from build123d import *

# Parameters (mm, degrees)
BOSS_EXTRUDE1_DEPTH = 50.1015


with BuildPart() as part:
    # Sketch1 → Boss-Extrude1 (new, symmetric)
    with BuildSketch(Plane(origin=(0, 0, 0), x_dir=(1, 0, 0), z_dir=(0, 1, 0))):
        Polygon((2.886751346, 0), (1.443375673, 2.5), (-1.443375673, 2.5), (-2.886751346, 0), (-1.443375673, -2.5), (1.443375673, -2.5), align=None)
    extrude(amount=BOSS_EXTRUDE1_DEPTH, both=True)

    # Sketch3 → M3x0.5 Tapped Hole1 (revolve, cut)
    with BuildSketch(Plane(origin=(0, 50.1015, 0), x_dir=(0, 0, 1), z_dir=(1, 0, 0))):
        Polygon((0, 0), (0, 10.276075774), (1.25, 9.525), (1.25, 0), align=None)
    m3x0_5_tapped_hole1 = revolve(axis=Axis((0, 56.4515, 0), (0, -1, 0)), mode=Mode.SUBTRACT)

    # Mirror1: M3x0.5 Tapped Hole1 across plane
    add(m3x0_5_tapped_hole1.mirror(Plane.ZX), mode=Mode.SUBTRACT)


solid = part.part
Work out the finished part from the listing and answer in its coordinate system (mm). A direction names the side the tool comes from. Round coordinates to 2 decimals unless told otherwise and drop trailing zeros. Write each loop counter-clockwise with the first axis right and the second up, starting at its lowest first coordinate (ties: lowest second). Pieces come first, ordered by that corner, then holes. Notation, with made-up numbers: (26.25, 78.5) -> (60.25, 78.5) arc R15 cw to (60.25, 88.5) -> close; hole circle Ø1 at (52, 11). An arc over 180 degrees is marked (long way). Answer as CSV lines item,"result". Start each with the question number.
(1) The part is cut by section A-A, the plane y = 44. Give the vertices of the cut face in (x, z).
(2) The mould has two halves that part along Z. Classify faces 1 (the conical face through (0.212, 39.956, -0.047)), 2 (the cylindrical face through (1.22, 45.41, -0.27)), 3 (the flat face through (2.175, 0.701, -1.233)), 4 (the flat face through (0, 1, 2.5)): +Z half, -Z half, draft (parallel to the pull), parting line (faces both ways), or undercut.
(3) Each of these flat-tipped pins is pushed along its axis until it touches: pin 1 (3 mm diameter, centred on x = 0, z = 0, fed in from +Y); pin 2 (1 mm diameter, centred on y = 33.5, z = -1, fed in from -X); pin 3 (1 mm diameter, centred on x = -2, y = 1, fed in from -Z). Where does it stop, or does it pass through?
(4) A tool of negligible diameter and unlimited length cuts with its end or side. For faces 5 (the flat face through (2.155, 0.701, 1.267)), 6 (the cylindrical face through (1.22, -45.41, -0.27)), from which of +Z, -Z, +X, -X, +Y, -Y can it reach the whole face along a straight path? Write none if from no direction.
(5) Find the intervals of material crossed by probe 1 along X at (y, z) = (42, 0); probe 2 along Z at (x, y) = (0, -42.75); probe 3 along X at (y, z) = (45, -0.1), in increasing order.
(6) The part is cut by section B-B, the plane y = 31. Give the vertices of the cut face in (x, z), then the cut area to 3 significant figures.
Output values:
1,outline,"(-2.89, 0) -> (-1.44, -2.5) -> (1.44, -2.5) -> (2.89, 0) -> (1.44, 2.5) -> (-1.44, 2.5) -> close; hole circle Ø2.5 at (0, 0)"
2,face 1,"undercut"
2,face 2,"undercut"
2,face 3,"-Z half"
2,face 4,"+Z half"
3,pin 1,"stops at y = 50.1"
3,pin 2,"stops at x = -2.6"
3,pin 3,"stops at z = -2.4"
4,face 5,"+Z, +X, +Y, -Y"
4,face 6,"-Y"
5,probe 1,"x = -2.89 to -1.25, 1.25 to 2.89"
5,probe 2,"z = -2.5 to -1.25, 1.25 to 2.5"
5,probe 3,"x = -2.83 to -1.25, 1.25 to 2.83"
6,outline,"(-2.89, 0) -> (-1.44, -2.5) -> (1.44, -2.5) -> (2.89, 0) -> (1.44, 2.5) -> (-1.44, 2.5) -> close"
6,area,"21.7 mm²"
